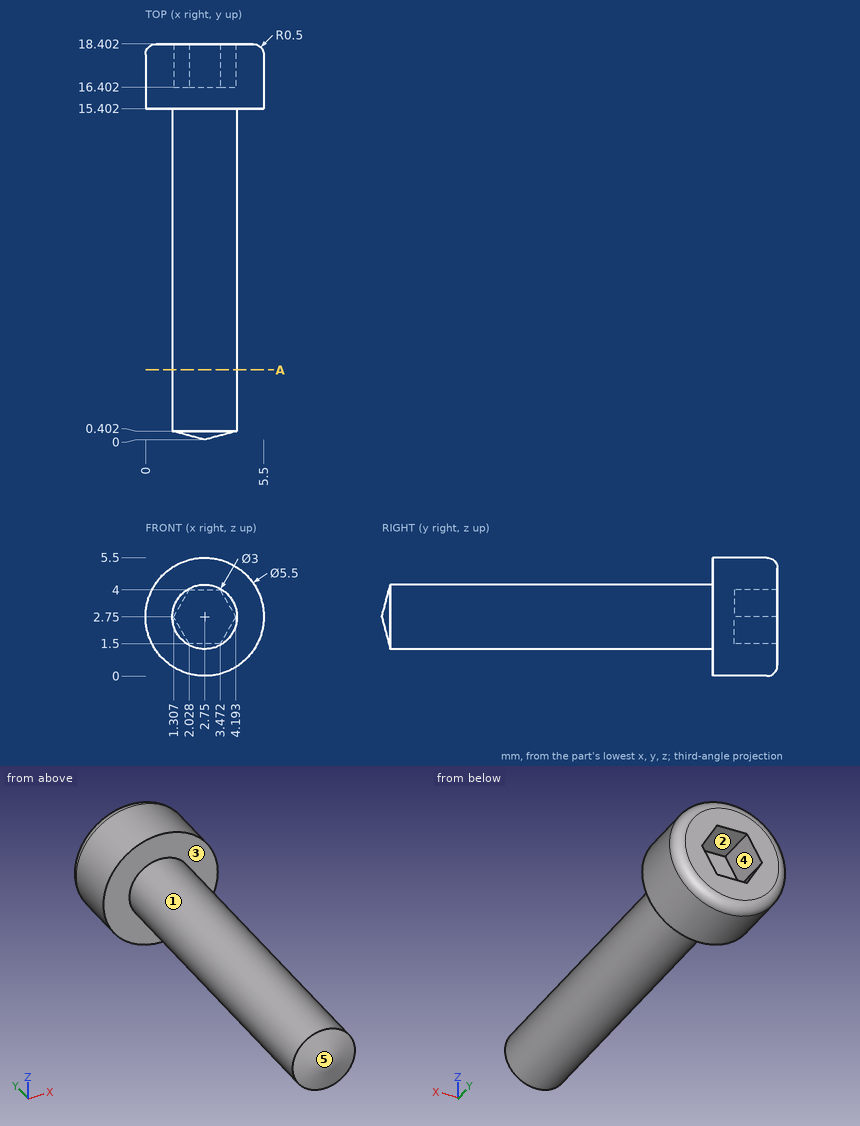
Input: dimensioned drawing with shaded views. Units: mm. Origin: part minimum x, y, z. A direction names the side the tool comes from. Coordinates: 2 decimals unless noted, no trailing zeros. Loops run counter-clockwise (first coordinate to the right, second up) from the corner with the lowest first, then second, coordinate; pieces in that order, holes last. Notation, with made-up numbers: (46.5, 82) - (88.5, 82) arc R19 ccw to (88.5, 117) - close; hole circle Ø11 at (64.5, -25.5). An arc over 180 degrees is marked (long way). One line per question, with ' | ' between items. Start each with the question number.
(1) Reachability of the marked faces 4 and 5 from +Z, -Z, +X, -X, +Y, -Y: full face, straight path, thin tool, end or side. Return the list, or none.
(2) First-contact query: pin 1 (1 mm diameter, centred on y = 9.5, z = 3, fed in from +X); pin 2 (3 mm diameter, centred on x = 1, y = 5, fed in from -Z); pin 3 (3 mm diameter, centred on x = 3, y = 12.5, fed in from +Z). Flat tips, straight axial feed; report the tip coordinate or a pass-through.
(3) Ray query, L1, parallel to X at y = 16.5, z = 1.65; L2, parallel to Z at x = 3.05, y = 17.25; L3, parallel to Y at x = 2.8, z = 0.6. Return the intervals inside material, ascending. Write a range as from..to.
(4) Cut plane A-A on y = 3.25. Output: boundary loops of the cut face in (x, z).
(5) Draft query along Z for the marked faces 1, 2 and 3. Return one class per face: +Z half, -Z half, draft (parallel to the pull), parting line (faces both ways), or undercut.
Here are the results:
1) face 4: +Y | face 5: -Y
2) pin 1: x = 4.25 | pin 2: z = 1.27 | pin 3: z = 4.25
3) L1: 0.23..1.94, 3.56..5.27 | L2: 0.02..1.5, 4..5.48 | L3: 15.4..18.4
4) outline: circle Ø3 at (2.75, 2.75)
5) face 1: parting line | face 2: undercut | face 3: draft
